Geometry: final body of the model. Coordinates: model frame, mm. Round coordinates to 2 decimals unless told otherwise and drop trailing zeros. Loops run counter-clockwise (first coordinate to the right, second up) from the corner with the lowest first, then second, coordinate; pieces in that order, holes last. Notation, with made-up numbers: (37, 63) -> (41, 63) arc R38 ccw to (41, 101) -> close; hole circle Ø6 at (28, -12.75). An arc over 180 degrees is marked (long way). Answer in a Markdown table with one row per item.
```python
from build123d import *

# Parameters (mm, degrees)
F0_W     = 3.3884318545
F0_H     = 5.3184241988
F1_DEPTH = 3.4
F2_R     = 1.6899494937
F3_SCALE = 0.125


with BuildPart() as f1:
    # F0 (on Front) → F1 (new body)
    with BuildSketch(Plane.XZ):
        Polygon((16.7311448604, 3.6973168608), (-58.6892813444, 3.6973168608), (-58.6892813444, 0), (13.3427130058, 0), (16.7311448604, 0), align=None)
        with Locations((15.0369289331, -2.6592120994)):
            Rectangle(F0_W, F0_H)
    extrude(amount=F1_DEPTH)

    # F2
    f2_edges = [f1.edges().sort_by_distance(p)[0] for p in [
        (-20.979068, -3.4, 3.697317),
        (-20.979068, 0, 3.697317),
        (-22.673284, -3.4, 0),
        (-22.673284, 0, 0),
    ]]
    fillet(f2_edges, radius=F2_R)


with BuildPart() as f1_1:
    # F3: moved
    add(f1.part.scale(F3_SCALE))


solid = f1_1.part
```
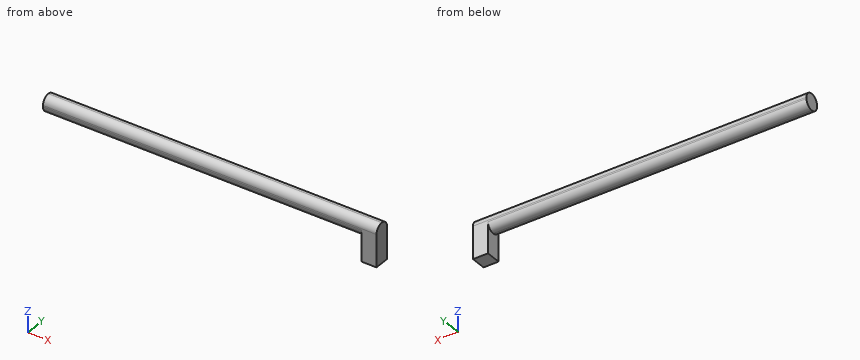
Item 1: Cut plane B-B (z = 0.1). Output: boundary loops of the cut face in (x, y) (3 decimals), then the cut area to 3 significant figures.
Answer:
| item | result |
|---|---|
| outline | (-7.336, -0.393) -> (1.668, -0.393) -> (1.668, -0.425) -> (2.091, -0.425) -> (2.091, 0) -> (1.668, 0) -> (1.668, -0.032) -> (-7.336, -0.032) -> close |
| area | 3.44 mm² |
Item 2: Cut plane C-C (y = -0.1). Output: boundary loops of the cut face in (x, z), then the cut area to 3 significant figures.
Answer:
| item | result |
|---|---|
| outline | (-7.34, 0.03) -> (1.67, 0.03) -> (1.67, -0.66) -> (2.09, -0.66) -> (2.09, 0.43) -> (-7.34, 0.43) -> close |
| area | 4.06 mm² |
Item 3: Line query: probe 1 along X at (y, z) = (-0.3, -0.4); probe 2 along Z at (x, y) = (0.25, -0.2); probe 3 along Z at (x, y) = (1.25, -0.3). Output: solid intervals per line, ascending. Write a range as [from, to].
Answer:
| item | result |
|---|---|
| probe 1 | x = [1.67, 2.09] |
| probe 2 | z = [0, 0.46] |
| probe 3 | z = [0.02, 0.44] |
